Model file for the job. Use its own axes, mm. Face numbers are marked on the shaded views. A direction names the side the tool comes from. Coordinates: 2 decimals unless noted, no trailing zeros. Write each loop counter-clockwise with the first axis right and the second up, starting at its lowest first coordinate (ties: lowest second). Pieces come first, ordered by that corner, then holes. Notation, with made-up numbers: M -15,84 L -2,84 A34 cw -2,119 Z; hole C 78.25,-20 d9. An arc over 180 degrees is marked long. Put each result on its own line as item: value. Start each with the question number.
Q1. Cut at D-D (y = 20.5). Write the cut outline in (x, z).
Q2. Cut at C-C (x = -8). Write the cut outline in (y, z).
Q3. Cut at B-B (z = 4). Write the cut outline in (x, y) (3 decimals), then the cut area to 3 significant figures.
Q4. Cut at A-A (y = 0). Write the cut outline in (x, z) (3 decimals).
Q5. Drill centre lines: line 1 along Y through (x, z) = (0, 10) (3 decimals); line 2 along X through (y, z) = (-0.5, -6); line 3 along Y through (x, z) = (-23.5, -20). Where is each one in solid material? Low to high.
Q6. Drop flat-ended pins along their axis: pin 1 (2 mm diameter, centred on x = 30.5, z = -6, fed in from -Y); pin 2 (4 mm diameter, centred on x = 43.5, z = 10, fed in from -Y); pin 3 (8 mm diameter, centred on x = 7.5, y = -20.5, fed in from -Z); pin 4 (2 mm diameter, centred on x = -11.5, z = 20, fed in from +Y). Give the stop position or say it passes through.
Q7. Which spindle directions (+Z, -Z, +X, -X, +Y, -Y) get a long thin tool onto all of the face, cutting with end or side? Do the marked faces 1 and 2. Say none if no direction does.
Q8. Pull direction Y, two halves, no side cores. Call the marked faces 3, 4, 5 and 6: pulls with the +Y half, pulls with the -Y half, needs draft (parallel to the pull), parting line crosses it, or undercut.
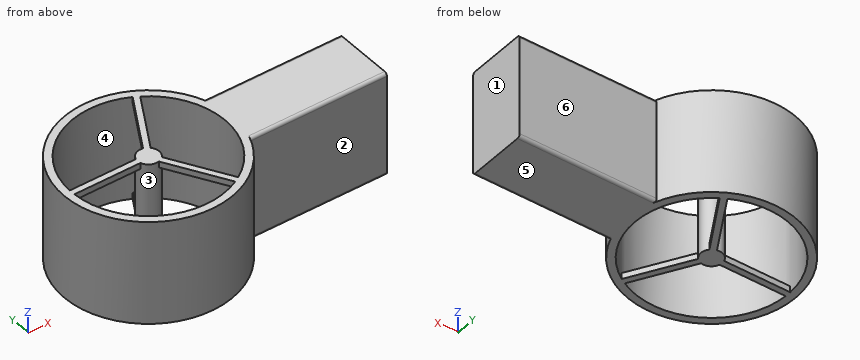
```python
from build123d import *

# Parameters (mm, degrees)
SKETCH1_R           = 34.925
BOSS_EXTRUDE1_DEPTH = 21.59
SKETCH2_W           = 43.18
SKETCH2_H           = 25.6
BOSS_EXTRUDE2_DEPTH = 89.408
SKETCH3_R           = 31.75
CUT_EXTRUDE1_DEPTH  = 106.252356216
SKETCH4_R           = 4.450657561
BOSS_EXTRUDE3_DEPTH = 43.18
EXTRUDE_THIN1_START = -2.54
EXTRUDE_THIN1_DEPTH = 2.54
FILLET1_R           = 1.27


# Read off the part's stored shape, not the designer's step: Extrude-Thin1
with BuildPart() as part:
    # Sketch1 → Boss-Extrude1 (new, symmetric)
    with BuildSketch(Plane.XY):
        Circle(SKETCH1_R)
    extrude(amount=BOSS_EXTRUDE1_DEPTH, both=True)

    # Sketch2 → Boss-Extrude2 (add)
    with BuildSketch(Plane(origin=(0, 0, 0), x_dir=(0, 0, -1), z_dir=(1, 0, 0))):
        Rectangle(SKETCH2_W, SKETCH2_H)
    extrude(amount=BOSS_EXTRUDE2_DEPTH)

    # Sketch3 → Cut-Extrude1 (cut, through all)
    with BuildSketch(Plane.XY.offset(21.59)):
        Circle(SKETCH3_R)
    extrude(amount=-CUT_EXTRUDE1_DEPTH, mode=Mode.SUBTRACT)



with BuildPart() as body_2:
    # Sketch4 → Boss-Extrude3 (new body)
    with BuildSketch(Plane.XY.offset(21.59)):
        Circle(SKETCH4_R)
    extrude(amount=-BOSS_EXTRUDE3_DEPTH)


with BuildPart() as part_1:
    add(part.part)

    add(body_2.part)  # Extrude-Thin1 merges body 2
    # Extrude-Thin1 outline → Extrude-Thin1 (add)
    with BuildSketch(Plane.XY.offset(21.59).offset(EXTRUDE_THIN1_START)):
        with BuildLine():
            ThreePointArc((-31.724589832, 1.27), (-31.75, 0), (-31.724589832, -1.27))
            Line((-31.724589832, -1.27), (-4.265612819, -1.27))
            ThreePointArc((-4.265612819, -1.27), (-4.450657561, 0), (-4.265612819, 1.27))
            Line((-4.265612819, 1.27), (-31.724589832, 1.27))
        make_face()
        with BuildLine():
            Line((1.032954147, -4.329129064), (14.762442653, -28.109300719))
            ThreePointArc((14.762442653, -28.109300719), (15.875, -27.49630657), (16.962147179, -26.839300719))
            Line((16.962147179, -26.839300719), (3.232658672, -3.059129064))
            ThreePointArc((3.232658672, -3.059129064), (2.225328781, -3.854382511), (1.032954147, -4.329129064))
        make_face()
        with BuildLine():
            ThreePointArc((16.962147179, 26.839300719), (15.875, 27.49630657), (14.762442653, 28.109300719))
            Line((14.762442653, 28.109300719), (1.032954147, 4.329129064))
            ThreePointArc((1.032954147, 4.329129064), (2.225328781, 3.854382511), (3.232658672, 3.059129064))
            Line((3.232658672, 3.059129064), (16.962147179, 26.839300719))
        make_face()
    extrude_thin1 = extrude(amount=EXTRUDE_THIN1_DEPTH)

    # Mirror1: Extrude-Thin1 across plane
    add(extrude_thin1.mirror(Plane.XY))

    # Fillet1
    fillet1_edges = [part_1.edges().sort_by_distance(p)[0] for p in [
        (60.951427681, 12.8, -21.59),
        (60.951427681, -12.8, 21.59),
        (60.951427681, -12.8, -21.59),
        (60.951427681, 12.8, 21.59),
    ]]
    fillet(fillet1_edges, radius=FILLET1_R)


solid = part_1.part
```
Computed values:
1. outline: M -28.28,-21.59 L -24.24,-21.59 L -24.24,21.59 L -28.28,21.59 Z; M 10.37,-21.59 L 13.3,-21.59 L 13.3,-19.05 L 10.37,-19.05 Z; M 10.37,19.05 L 13.3,19.05 L 13.3,21.59 L 10.37,21.59 Z; M 24.24,-21.59 L 28.28,-21.59 L 28.28,21.59 L 24.24,21.59 Z
2. outline: M -34,-21.59 L -30.73,-21.59 L -30.73,21.59 L -34,21.59 Z; M -1.27,-21.59 L 1.27,-21.59 L 1.27,-19.05 L -1.27,-19.05 Z; M -1.27,19.05 L 1.27,19.05 L 1.27,21.59 L -1.27,21.59 Z; M 30.73,-21.59 L 34,-21.59 L 34,21.59 L 30.73,21.59 Z
3. outline: C 0,0 d8.901; M 32.495,-12.8 L 89.408,-12.8 L 89.408,12.8 L 32.495,12.8 A34.925 ccw long Z; hole C 0,0 d63.5
3. area: 2,140 mm2
4. outline: M -34.925,-21.59 L 4.451,-21.59 L 4.451,21.59 L -34.925,21.59 Z; M 31.75,-21.59 L 89.408,-21.59 L 89.408,21.59 L 31.75,21.59 Z; hole M -31.75,-19.05 L -4.451,-19.05 L -4.451,19.05 L -31.75,19.05 Z
5. line 1: -34.925 to -31.75, -4.451 to 4.451, 31.75 to 34.925
5. line 2: -34.92 to -31.75, -4.42 to 4.42, 31.75 to 89.41
5. line 3: -25.84 to -21.35, -1.27 to 1.27, 21.35 to 25.84
6. pin 1: y = -18.7
6. pin 2: y = -12.8
6. pin 3: z = -21.59
6. pin 4: y = 33.31
7. face 1: +Z, -Z, +X, +Y, -Y
7. face 2: +Z, -Z, +X, -Y
8. face 3: undercut
8. face 4: undercut
8. face 5: needs draft
8. face 6: pulls with the +Y half
